CAD build for the part. Positions are in the model's coordinates, mm. A direction names the side the tool comes from. Coordinates: 2 decimals unless noted, no trailing zeros. Loops run counter-clockwise (first coordinate to the right, second up) from the corner with the lowest first, then second, coordinate; pieces in that order, holes last. Notation, with made-up numbers: (-29, 36) -> (-20, 36) arc R26 cw to (-20, 57) -> close; hole circle Ø11 at (-12.5, 32.5). An arc over 180 degrees is marked (long way). Return JSON: item names as keys, results as strings. Group by question number.
(1) Saw through at C-C on x = -100. Write the cut outline in (y, z), then the cut area to 3 significant figures.
(2) Mould opens along Z. For faces 6 (the face through (-95, 5, 30)), 7 (the face through (-104, 54, 75)) say: pulls with the +Z half, pulls with the -Z half, needs draft (parallel to the pull), parting line crosses it, or undercut.
(3) Saw through at D-D on z = 66.5. Write the cut outline in (x, y).
(4) Saw through at A-A on z = 25. Write the cut outline in (x, y).
(5) Probe L1, parallel to Z at x = -104, y = 24.5; L2, parallel to Z at x = -95, y = 3; L3, parallel to Y at x = -93.5, z = 41.5. List the from-to ranges inside material, lowest first.
(6) Saw through at B-B on y = 27. Write the cut outline in (x, z).
(7) Flat gauge pins, fed straight in: pin 1 Ø6 at (x, z) = (-73.5, 48.5) entering from +Y; pin 2 Ø4 at (x, y) = (-75, 30) entering from +Z; pin 3 Ø9 at (y, z) = (55, 26.5) entering from -X. Where does each tip first touch, or does it go through?
(8) Tool access for faces 1 (the face through (-95, 54, 71)), 2 (the face through (-95, 40, 67)), 3 (the face through (-80, 25, 16)), 4 (the face through (-105, 5, 25)), 5 (the face through (-15, 38, 47.5)): list every direction of +Z, -Z, +X, -X, +Y, -Y with a clear straight run to the whole face (end or side of a thin tool).
Autodesk Inventor part; units mm, degrees
ref_plane "YZ Plane" through (0, 0, 0) normal (1, 0, 0) x (0, 1, 0)
ref_plane "XZ Plane" through (0, 0, 0) normal (0, 1, 0) x (-1, 0, 0)
ref_plane "XY Plane" through (0, 0, 0) normal (0, 0, 1) x (1, 0, 0)
sketch "Sketch1" plane through (0, 0, 0) normal (0, 1, 0) x (-1, 0, 0)
  line L0 (-10, -55) -> (-160, -55)
  line L1 (-160, -55) -> (-160, -45)
  line L2 (-160, -45) -> (-10, -45)
  line L3 (-10, -45) -> (-10, -55)
  line L4 (10, -55) -> (80, -55)
  line L5 (80, -55) -> (80, -90)
  line L6 (80, -90) -> (110, -90)
  line L7 (110, -90) -> (110, -10)
  line L8 (110, -10) -> (80, -10)
  line L9 (80, -10) -> (80, -45)
  line L10 (80, -45) -> (10, -45)
  line L11 (10, -45) -> (10, -55)
  line L12 (0, -122.2654) -> (0, -189.4683)
  line L13 (-10, 55) -> (-10, 45)
  line L14 (10, 55) -> (10, 45)
  line L15 (80, 10) -> (110, 10)
  line L16 (10, 45) -> (80, 45)
  line L17 (80, 45) -> (80, 10)
  line L18 (80, 55) -> (10, 55)
  line L19 (80, 90) -> (80, 55)
  line L20 (110, 10) -> (110, 90)
  line L21 (110, 90) -> (80, 90)
  line L22 (-160, 55) -> (-10, 55)
  line L23 (-160, 45) -> (-160, 55)
  line L24 (-10, 45) -> (-160, 45)
  point P0 (0, 0)
  dimension "d0" = 10
  dimension "d1" = 80
  dimension "d2" = 10
  dimension "d4" = 30
  dimension "d5" = 30
  dimension "d6" = 35
  dimension "d7" = 35
  dimension "d8" = 45
  dimension "d9" = 10
  dimension "d10" = 10
  dimension "d11" = 150
  dimension "d12" = 100
  dimension "d13" = 0
  dimension "d16" = 100
extrude "Extrusion1" add sketch "Sketch1" along normal blind 50
sketch "Sketch2" plane through (160, 0, 55) normal (1, 0, 0) x (0, 0, -1)
  line L0 (2.5, 40) -> (7.5, 40)
  line L1 (7.5, 40) -> (7.5, 35)
  line L2 (7.5, 35) -> (2.5, 35)
  line L3 (2.5, 35) -> (2.5, 40)
  line L4 (0, 50) -> (10, 50)
  line L5 (10, 0) -> (10, 50)
  line L6 (2.5, 15) -> (7.5, 15)
  line L7 (7.5, 15) -> (7.5, 10)
  line L8 (7.5, 10) -> (2.5, 10)
  line L9 (2.5, 10) -> (2.5, 15)
  line L10 (102.5, 40) -> (107.5, 40)
  line L11 (107.5, 40) -> (107.5, 35)
  line L12 (107.5, 35) -> (102.5, 35)
  line L13 (102.5, 35) -> (102.5, 40)
  line L14 (102.5, 15) -> (107.5, 15)
  line L15 (107.5, 15) -> (107.5, 10)
  line L16 (107.5, 10) -> (102.5, 10)
  line L17 (102.5, 10) -> (102.5, 15)
  point P0 (55, 0)
  dimension "d23" = 10
  dimension "d24" = 5
  dimension "d25" = 2.5
  dimension "d26" = 5
  dimension "d29" = 25
  dimension "d32" = 100
extrude "Extrusion2" cut sketch "Sketch2" against normal blind 200
sketch "Sketch3" plane through (0, 50, 0) normal (0, 1, 0) x (1, 0, 0)
  line L0 (-105, -20) -> (-85, -20)
  line L1 (-85, -20) -> (-85, -30)
  line L2 (-85, -30) -> (-105, -30)
  line L3 (-105, -30) -> (-105, -20)
  line L4 (-110, -10) -> (-110, -90)
  line L5 (-105, -70) -> (-85, -70)
  line L6 (-85, -70) -> (-85, -80)
  line L7 (-85, -80) -> (-105, -80)
  line L8 (-105, -80) -> (-105, -70)
  line L9 (-105, 80) -> (-85, 80)
  line L10 (-85, 80) -> (-85, 70)
  line L11 (-85, 70) -> (-105, 70)
  line L12 (-105, 70) -> (-105, 80)
  line L13 (-105, 30) -> (-85, 30)
  line L14 (-85, 30) -> (-85, 20)
  line L15 (-85, 20) -> (-105, 20)
  line L16 (-105, 20) -> (-105, 30)
  point P0 (0, 0)
  dimension "d37" = 20
  dimension "d38" = 10
  dimension "d39" = 20
  dimension "d40" = 85
  dimension "d43" = 50
  dimension "d46" = 100
extrude "Extrusion3" add sketch "Sketch3" along normal blind 8
sketch "Sketch4" plane through (0, 0, 0) normal (0, -1, 0) x (1, 0, 0)
  line L0 (-105, -70) -> (-85, -70)
  line L1 (-85, -70) -> (-85, -80)
  line L2 (-85, -80) -> (-105, -80)
  line L3 (-105, -80) -> (-105, -70)
  line L4 (-105, -20) -> (-85, -20)
  line L5 (-85, -20) -> (-85, -30)
  line L6 (-85, -30) -> (-105, -30)
  line L7 (-105, -30) -> (-105, -20)
  line L8 (-105, 30) -> (-85, 30)
  line L9 (-85, 30) -> (-85, 20)
  line L10 (-85, 20) -> (-105, 20)
  line L11 (-105, 20) -> (-105, 30)
  line L12 (-105, 80) -> (-85, 80)
  line L13 (-85, 80) -> (-85, 70)
  line L14 (-85, 70) -> (-105, 70)
  line L15 (-105, 70) -> (-105, 80)
  line L16 (-85, 80) -> (-105, 80)
  line L17 (-105, 80) -> (-105, 70)
  line L18 (-105, 70) -> (-85, 70)
  line L19 (-85, 70) -> (-85, 80)
  line L20 (-85, 30) -> (-105, 30)
  line L21 (-105, 30) -> (-105, 20)
  line L22 (-105, 20) -> (-85, 20)
  line L23 (-85, 20) -> (-85, 30)
  line L24 (-85, -20) -> (-105, -20)
  line L25 (-105, -20) -> (-105, -30)
  line L26 (-105, -30) -> (-85, -30)
  line L27 (-85, -30) -> (-85, -20)
  line L28 (-85, -70) -> (-105, -70)
  line L29 (-105, -70) -> (-105, -80)
  line L30 (-105, -80) -> (-85, -80)
  line L31 (-85, -80) -> (-85, -70)
  point P0 (0, 0)
extrude "Extrusion4" cut sketch "Sketch4" against normal blind 10
sketch "Sketch5" plane through (10, 0, 55) normal (0, 0, 1) x (1, 0, 0)
  line L0 (0, 0) -> (0, 50)
  line L1 (0, 50) -> (150, 50)
  line L2 (150, 0) -> (150, 50)
  line L3 (0, 0) -> (150, 0)
  line L4 (0, 35) -> (0, 40)
  line L5 (150, 35) -> (0, 35)
  line L6 (150, 40) -> (150, 35)
  line L7 (150, 40) -> (0, 40)
  line L8 (0, 10) -> (0, 15)
  line L9 (150, 10) -> (0, 10)
  line L10 (150, 15) -> (150, 10)
  line L11 (150, 15) -> (0, 15)
  line L12 (10, 40) -> (140, 40)
  line L13 (140, 40) -> (140, 35)
  line L14 (140, 35) -> (10, 35)
  line L15 (10, 35) -> (10, 40)
  line L16 (10, 15) -> (140, 15)
  line L17 (140, 15) -> (140, 10)
  line L18 (140, 10) -> (10, 10)
  line L19 (10, 10) -> (10, 15)
  point P0 (-10, 0)
  point P1 (10, 10)
  dimension "d53" = 10
  dimension "d54" = 10
  dimension "d55" = 10
  dimension "d56" = 10
extrude "Extrusion5" add sketch "Sketch5" against normal blind 10 contours L19 L11 L17 L9 | L15 L7 L13 L5
sketch "Sketch6" plane through (160, 0, -55) normal (0, 0, -1) x (-1, 0, 0)
  line L0 (150, 40) -> (150, 35)
  line L1 (0, 40) -> (150, 40)
  line L2 (0, 35) -> (0, 40)
  line L3 (0, 35) -> (150, 35)
  line L4 (150, 15) -> (150, 10)
  line L5 (0, 15) -> (150, 15)
  line L6 (0, 10) -> (0, 15)
  line L7 (0, 10) -> (150, 10)
  line L8 (10, 40) -> (140, 40)
  line L9 (140, 40) -> (140, 35)
  line L10 (140, 35) -> (10, 35)
  line L11 (10, 35) -> (10, 40)
  line L12 (10, 15) -> (140, 15)
  line L13 (140, 15) -> (140, 10)
  line L14 (140, 10) -> (10, 10)
  line L15 (10, 10) -> (10, 15)
  point P0 (160, 0)
  point P1 (140, 37.5)
  point P2 (10, 10)
  dimension "d59" = 10
  dimension "d60" = 10
  dimension "d61" = 10
  dimension "d62" = 10
extrude "Extrusion6" add sketch "Sketch6" against normal blind 10 contours L9 L3 L11 L1 | L13 L7 L15 L5
sketch "Sketch7" plane through (0, 58, 0) normal (0, 1, 0) x (1, 0, 0)
  line L0 (-105, -80) -> (-85, -80)
  line L1 (-85, -80) -> (-85, -70)
  line L2 (-85, -70) -> (-105, -70)
  line L3 (-105, -70) -> (-105, -80)
  line L4 (-105, -30) -> (-85, -30)
  line L5 (-85, -30) -> (-85, -20)
  line L6 (-85, -20) -> (-105, -20)
  line L7 (-105, -20) -> (-105, -30)
  line L8 (-105, 20) -> (-85, 20)
  line L9 (-85, 20) -> (-85, 30)
  line L10 (-85, 30) -> (-105, 30)
  line L11 (-105, 30) -> (-105, 20)
  line L12 (-105, 70) -> (-85, 70)
  line L13 (-85, 70) -> (-85, 80)
  line L14 (-85, 80) -> (-105, 80)
  line L15 (-105, 80) -> (-105, 70)
  line L16 (-104, -79) -> (-86, -79)
  line L17 (-86, -79) -> (-86, -71)
  line L18 (-86, -71) -> (-104, -71)
  line L19 (-104, -71) -> (-104, -79)
  line L20 (-86, -21) -> (-104, -21)
  line L21 (-104, -21) -> (-104, -29)
  line L22 (-104, -29) -> (-86, -29)
  line L23 (-86, -29) -> (-86, -21)
  line L24 (-86, 29) -> (-104, 29)
  line L25 (-104, 29) -> (-104, 21)
  line L26 (-104, 21) -> (-86, 21)
  line L27 (-86, 21) -> (-86, 29)
  line L28 (-86, 79) -> (-104, 79)
  line L29 (-104, 79) -> (-104, 71)
  line L30 (-104, 71) -> (-86, 71)
  line L31 (-86, 71) -> (-86, 79)
  line L32 (-105, -80) -> (-85, -80)
  line L33 (-85, -80) -> (-85, -70)
  line L34 (-85, -70) -> (-105, -70)
  line L35 (-105, -70) -> (-105, -80)
  line L36 (-105, -30) -> (-85, -30)
  line L37 (-85, -30) -> (-85, -20)
  line L38 (-85, -20) -> (-105, -20)
  line L39 (-105, -20) -> (-105, -30)
  line L40 (-105, 20) -> (-85, 20)
  line L41 (-85, 20) -> (-85, 30)
  line L42 (-85, 30) -> (-105, 30)
  line L43 (-105, 30) -> (-105, 20)
  line L44 (-105, 70) -> (-85, 70)
  line L45 (-85, 70) -> (-85, 80)
  line L46 (-85, 80) -> (-105, 80)
  line L47 (-105, 80) -> (-105, 70)
  point P0 (0, 0)
  dimension "d65" = 1
  dimension "d66" = 1
  dimension "d67" = 1
  dimension "d68" = 1
  dimension "d71" = 50
  dimension "d74" = 100
extrude "Extrusion7" cut sketch "Sketch7" against normal blind 8
sketch "Sketch8" plane through (-80, 0, 55) normal (0, 0, 1) x (1, 0, 0)
  line L0 (70, 40) -> (70, 35)
  line L1 (70, 40) -> (40, 40)
  line L2 (40, 40) -> (40, 35)
  line L3 (70, 35) -> (40, 35)
  line L4 (70, 15) -> (70, 10)
  line L5 (70, 15) -> (40, 15)
  line L6 (40, 15) -> (40, 10)
  line L7 (70, 10) -> (40, 10)
  line L8 (40, 40) -> (60, 40)
  line L9 (60, 40) -> (60, 35)
  line L10 (60, 35) -> (40, 35)
  line L11 (40, 35) -> (40, 40)
  line L12 (40, 15) -> (60, 15)
  line L13 (60, 15) -> (60, 10)
  line L14 (60, 10) -> (40, 10)
  line L15 (40, 10) -> (40, 15)
  point P0 (80, 0)
  point P1 (60, 15)
  point P2 (60, 40)
  dimension "d79" = 10
  dimension "d80" = 10
extrude "Extrusion8" add sketch "Sketch8" against normal blind 10 contours L9 L3 L2 L1 | L13 L7 L6 L5
sketch "Sketch9" plane through (-10, 0, -55) normal (0, 0, -1) x (-1, 0, 0)
  line L0 (0, 35) -> (0, 40)
  line L1 (0, 35) -> (30, 35)
  line L2 (30, 35) -> (30, 40)
  line L3 (0, 40) -> (30, 40)
  line L4 (0, 10) -> (0, 15)
  line L5 (0, 10) -> (30, 10)
  line L6 (30, 10) -> (30, 15)
  line L7 (0, 15) -> (30, 15)
  line L8 (30, 40) -> (10, 40)
  line L9 (10, 40) -> (10, 10)
  line L10 (10, 10) -> (30, 10)
  line L11 (30, 10) -> (30, 40)
  point P0 (-10, 0)
  point P1 (0, 37.5)
  dimension "d83" = 10
extrude "Extrusion9" add sketch "Sketch9" against normal blind 10 contours L9 L3 L2 L1 | L1 L11 L7 L9 | L7 L6 L5 L9
sketch "Sketch10" plane through (0, 58, 0) normal (0, 1, 0) x (1, 0, 0)
  line L0 (-140, 100) -> (-140, 0)
  line L1 (-140, 0) -> (0, 0)
  line L2 (0, 0) -> (0, -100)
  line L3 (0, -100) -> (180, -100)
  line L4 (180, -100) -> (180, 100)
  line L5 (180, 100) -> (-140, 100)
  dimension "d86" = 100
  dimension "d87" = 320
  dimension "d88" = 200
  dimension "d89" = 180
extrude "Extrusion10" cut sketch "Sketch10" against normal through all
sketch "Sketch11" plane through (-80, 0, 90) normal (1, 0, 0) x (0, 0, -1)
  line L0 (0, 0) -> (35, 0)
  line L1 (35, 0) -> (35, 50)
  line L2 (0, 50) -> (35, 50)
  line L3 (0, 0) -> (0, 50)
  line L4 (45, 0) -> (80, 0)
  line L5 (80, 0) -> (80, 50)
  line L6 (45, 50) -> (80, 50)
  line L7 (45, 0) -> (45, 50)
  line L8 (35, 40) -> (10, 40)
  line L9 (10, 40) -> (10, 10)
  line L10 (10, 10) -> (35, 10)
  line L11 (35, 10) -> (35, 40)
  line L12 (45, 40) -> (70, 40)
  line L13 (70, 40) -> (70, 10)
  line L14 (70, 10) -> (45, 10)
  line L15 (45, 10) -> (45, 40)
  point P0 (90, 0)
  point P1 (17.5, 0)
  point P2 (35, 10)
  dimension "d92" = 25
  dimension "d93" = 25
  dimension "d94" = 30
  dimension "d95" = 10
extrude "Extrusion11" cut sketch "Sketch11" against normal blind 30 contours L10 L9 L8 L1 | L7 L12 L13 L14
properties part number "Hurdle Split"
Geometry results:
{
 "1": {"outline": "(0, 10) -> (50, 10) -> (50, 21) -> (58, 21) -> (58, 29) -> (50, 29) -> (50, 71) -> (58, 71) -> (58, 79) -> (50, 79) -> (50, 90) -> (0, 90) -> (0, 80) -> (40, 80) -> (40, 55) -> (10, 55) -> (10, 70) -> (0, 70) -> (0, 30) -> (10, 30) -> (10, 45) -> (40, 45) -> (40, 20) -> (0, 20) -> close", "area": "2,430 mm²"},
 "2": {"face 6": "undercut", "face 7": "needs draft"},
 "3": {"outline": "(-110, 0) -> (-80, 0) -> (-80, 10) -> (-110, 10) -> close; (-110, 40) -> (-80, 40) -> (-80, 50) -> (-110, 50) -> close"},
 "4": {"outline": "(-110, 0) -> (-105, 0) -> (-105, 10) -> (-110, 10) -> close; (-110, 40) -> (-80, 40) -> (-80, 50) -> (-86, 50) -> (-86, 58) -> (-104, 58) -> (-104, 50) -> (-110, 50) -> close; (-85, 0) -> (-80, 0) -> (-80, 10) -> (-85, 10) -> close"},
 "5": {"L1": "10 to 20, 45 to 55, 80 to 90", "L2": "10 to 20, 30 to 70, 80 to 90", "L3": "0 to 10, 40 to 50"},
 "6": {"outline": "(-110, 10) -> (-80, 10) -> (-80, 20) -> (-110, 20) -> close; (-110, 45) -> (-10, 45) -> (-10, 55) -> (-110, 55) -> close; (-110, 80) -> (-80, 80) -> (-80, 90) -> (-110, 90) -> close"},
 "7": {"pin 1": "y = 50", "pin 2": "z = 55", "pin 3": "x = -104"},
 "8": {"face 1": "+X, -X, +Y", "face 2": "+X, -X", "face 3": "-Z, +X, +Y, -Y", "face 4": "-Y", "face 5": "+X"}
}
